from build123d import *

# Parameters (mm, degrees)
SKETCH1_W           = 15
SKETCH1_H           = 12.8
BOSS_EXTRUDE1_DEPTH = 1.7
SKETCH1_3_W         = 2
SKETCH1_3_H         = 1.2
BOSS_EXTRUDE2_DEPTH = 0.5
SKETCH1_4_R         = 0.35
CUT_EXTRUDE1_DEPTH  = 11.004998751


with BuildPart() as part:
    # Sketch1 → Boss-Extrude1 (new body)
    with BuildSketch(Plane.XY):
        Rectangle(SKETCH1_W, SKETCH1_H)
    extrude(amount=BOSS_EXTRUDE1_DEPTH)

    # Sketch1_3 → Boss-Extrude2 (add)
    with BuildSketch(Plane.XY):
        with Locations((-2, 0)):
            Rectangle(SKETCH1_3_W, SKETCH1_3_H)
        with Locations((-6, 0)):
            Rectangle(SKETCH1_3_W, SKETCH1_3_H)
        with Locations((2, 0)):
            Rectangle(SKETCH1_3_W, SKETCH1_3_H)
        with Locations((6, 0)):
            Rectangle(SKETCH1_3_W, SKETCH1_3_H)
    extrude(amount=-BOSS_EXTRUDE2_DEPTH)

    # Sketch1_4 → Cut-Extrude1 (cut, through all)
    with BuildSketch(Plane.XY):
        with Locations((-6.5, 5.7)):
            Circle(SKETCH1_4_R)
        with Locations((-3.9, 5.7)):
            Circle(SKETCH1_4_R)
        with Locations((-1.3, 5.7)):
            Circle(SKETCH1_4_R)
        with Locations((1.3, 5.7)):
            Circle(SKETCH1_4_R)
        with Locations((3.9, 5.7)):
            Circle(SKETCH1_4_R)
        with Locations((6.5, 5.7)):
            Circle(SKETCH1_4_R)
        with Locations(Location((-1.3, -5.7, 0), (0, 0, 180))):
            Circle(SKETCH1_4_R)
        with Locations(Location((6.5, -5.7, 0), (0, 0, 180))):
            Circle(SKETCH1_4_R)
        with Locations(Location((3.9, -5.7, 0), (0, 0, 180))):
            Circle(SKETCH1_4_R)
        with Locations(Location((1.3, -5.7, 0), (0, 0, 180))):
            Circle(SKETCH1_4_R)
        with Locations(Location((-3.9, -5.7, 0), (0, 0, 180))):
            Circle(SKETCH1_4_R)
        with Locations(Location((-6.5, -5.7, 0), (0, 0, 180))):
            Circle(SKETCH1_4_R)
    extrude(amount=CUT_EXTRUDE1_DEPTH, mode=Mode.SUBTRACT)


solid = part.part
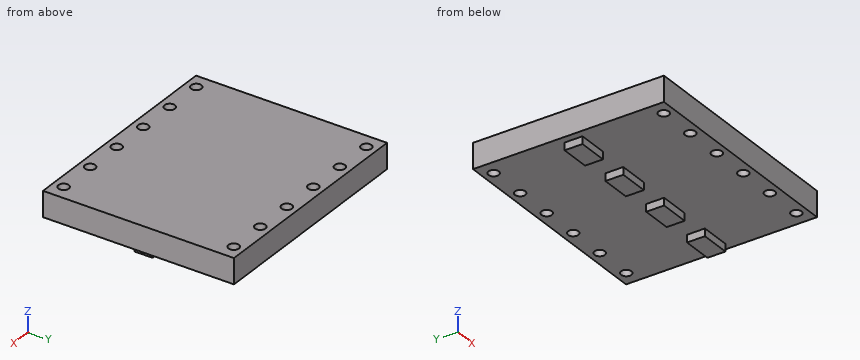
Design review of the part built by this model. Coordinates are the model's own, in mm. Round coordinates to 2 decimals unless told otherwise and drop trailing zeros. Write each loop counter-clockwise with the first axis right and the second up, starting at its lowest first coordinate (ties: lowest second). Pieces come first, ordered by that corner, then holes. Notation, with made-up numbers: (43, -16.5) -> (100, -16.5) arc R26 ccw to (100, 17.5) -> close; hole circle Ø11 at (6, 36.5). An arc over 180 degrees is marked (long way). One line per item, written item: value. Start each with the question number.
Q1. To check wall thickness, follow probe 1 along Y at (x, z) = (1.3, 0.85); probe 2 along Z at (x, y) = (-7, -1). State the ranges of each line that lie inside material, in increasing order.
Q2. Insertion check: P1, Ø1.5, axis at x = 4.5, y = 2.5, coming from the -Z side; P2, Ø5, axis at x = 5.5, y = 3, coming from the -Z side. Each pin has a flat end and moves straight along its axis. Give the tip position at first contact, or say it passes through.
Q3. Add section B-B (z = -0.2). Give the boundary of the cut face in (x, y).
Q4. Add section D-D (z = 1.15). State how many separate pieces and enclosed holes the cut face has, then the cut area to 3 significant figures.
Q5. Add section C-C (x = -3.9). Give the boundary of the cut face in (y, z), then the cut area to 3 significant figures.
Q6. Add section A-A (y = -5.7). Give the boundary of the cut face in (x, z), then the cut area to 3 significant figures.
Response:
1. probe 1: y = -6.4 to -6.05, -5.35 to 5.35, 6.05 to 6.4
1. probe 2: z = 0 to 1.7
2. P1: stops at z = 0
2. P2: stops at z = -0.5
3. outline: (-7, -0.6) -> (-5, -0.6) -> (-5, 0.6) -> (-7, 0.6) -> close; (-3, -0.6) -> (-1, -0.6) -> (-1, 0.6) -> (-3, 0.6) -> close; (1, -0.6) -> (3, -0.6) -> (3, 0.6) -> (1, 0.6) -> close; (5, -0.6) -> (7, -0.6) -> (7, 0.6) -> (5, 0.6) -> close
4. separate pieces: 1
4. enclosed holes: 12
4. area: 187 mm^2
5. outline: (-6.4, 0) -> (-6.05, 0) -> (-6.05, 1.7) -> (-6.4, 1.7) -> close; (-5.35, 0) -> (5.35, 0) -> (5.35, 1.7) -> (-5.35, 1.7) -> close; (6.05, 0) -> (6.4, 0) -> (6.4, 1.7) -> (6.05, 1.7) -> close
5. area: 19.4 mm^2
6. outline: (-7.5, 0) -> (-6.85, 0) -> (-6.85, 1.7) -> (-7.5, 1.7) -> close; (-6.15, 0) -> (-4.25, 0) -> (-4.25, 1.7) -> (-6.15, 1.7) -> close; (-3.55, 0) -> (-1.65, 0) -> (-1.65, 1.7) -> (-3.55, 1.7) -> close; (-0.95, 0) -> (0.95, 0) -> (0.95, 1.7) -> (-0.95, 1.7) -> close; (1.65, 0) -> (3.55, 0) -> (3.55, 1.7) -> (1.65, 1.7) -> close; (4.25, 0) -> (6.15, 0) -> (6.15, 1.7) -> (4.25, 1.7) -> close; (6.85, 0) -> (7.5, 0) -> (7.5, 1.7) -> (6.85, 1.7) -> close
6. area: 18.4 mm^2
